```python
from build123d import *

# Parameters (mm, degrees)
SKETCH1_W           = 242
SKETCH1_H           = 13
SKETCH1_R           = 1.5
BOSS_EXTRUDE1_DEPTH = 2
CUT_EXTRUDE1_REACH  = 123.713
SKETCH2_W           = 30
SKETCH2_H           = 4
SKETCH3_W           = 242
SKETCH3_H           = 2
BOSS_EXTRUDE2_DEPTH = 15
CUT_EXTRUDE2_REACH  = 124.845
SKETCH4_R           = 1.5
FILLET1_R           = 12


with BuildPart() as part:
    # Sketch1 → Boss-Extrude1 (new body)
    with BuildSketch(Plane.XY):
        with Locations((0, -6.5)):
            Rectangle(SKETCH1_W, SKETCH1_H)
        with Locations((-114, -6.5)):
            Circle(SKETCH1_R, mode=Mode.SUBTRACT)
        with Locations((-44, -6.5)):
            Circle(SKETCH1_R, mode=Mode.SUBTRACT)
        with Locations((-24, -6.5)):
            Circle(SKETCH1_R, mode=Mode.SUBTRACT)
        with Locations((27, -6.5)):
            Circle(SKETCH1_R, mode=Mode.SUBTRACT)
        with Locations((97, -6.5)):
            Circle(SKETCH1_R, mode=Mode.SUBTRACT)
    extrude(amount=BOSS_EXTRUDE1_DEPTH)

    # Sketch2 → Cut-Extrude1 (cut, up to next)
    with BuildSketch(Plane.XY.offset(2), mode=Mode.PRIVATE) as cut_extrude1_sk1:
        with Locations((-3, -11)):
            Rectangle(SKETCH2_W, SKETCH2_H)
    cut_extrude1_tool1 = extrude(cut_extrude1_sk1.sketch, amount=-CUT_EXTRUDE1_REACH, mode=Mode.PRIVATE) & part.part
    add(cut_extrude1_tool1.solids().sort_by_distance((-3, -11, 2))[0], mode=Mode.SUBTRACT)

    # Sketch3 → Boss-Extrude2 (add)
    with BuildSketch(Plane.XY):
        with Locations((0, 1)):
            Rectangle(SKETCH3_W, SKETCH3_H)
    extrude(amount=BOSS_EXTRUDE2_DEPTH)

    # Sketch4 → Cut-Extrude2 (cut, up to next)
    with BuildSketch(Plane(origin=(0, 2, 0), x_dir=(1, 0, 0), z_dir=(0, 1, 0)), mode=Mode.PRIVATE) as cut_extrude2_sk1:
        with Locations(Location((-110, -7.5, 0), (0, 0, 270))):
            Circle(SKETCH4_R)
    cut_extrude2_tool1 = extrude(cut_extrude2_sk1.sketch, amount=-CUT_EXTRUDE2_REACH, mode=Mode.PRIVATE) & part.part
    # Sketch4 → Cut-Extrude2 (cut, up to next)
    with BuildSketch(Plane(origin=(0, 2, 0), x_dir=(1, 0, 0), z_dir=(0, 1, 0)), mode=Mode.PRIVATE) as cut_extrude2_sk2:
        with Locations(Location((-50, -7.5, 0), (0, 0, 270))):
            Circle(SKETCH4_R)
    cut_extrude2_tool2 = extrude(cut_extrude2_sk2.sketch, amount=-CUT_EXTRUDE2_REACH, mode=Mode.PRIVATE) & part.part
    # Sketch4 → Cut-Extrude2 (cut, up to next)
    with BuildSketch(Plane(origin=(0, 2, 0), x_dir=(1, 0, 0), z_dir=(0, 1, 0)), mode=Mode.PRIVATE) as cut_extrude2_sk3:
        with Locations(Location((45, -7.5, 0), (0, 0, 270))):
            Circle(SKETCH4_R)
    cut_extrude2_tool3 = extrude(cut_extrude2_sk3.sketch, amount=-CUT_EXTRUDE2_REACH, mode=Mode.PRIVATE) & part.part
    # Sketch4 → Cut-Extrude2 (cut, up to next)
    with BuildSketch(Plane(origin=(0, 2, 0), x_dir=(1, 0, 0), z_dir=(0, 1, 0)), mode=Mode.PRIVATE) as cut_extrude2_sk4:
        with Locations(Location((112, -7.5, 0), (0, 0, 270))):
            Circle(SKETCH4_R)
    cut_extrude2_tool4 = extrude(cut_extrude2_sk4.sketch, amount=-CUT_EXTRUDE2_REACH, mode=Mode.PRIVATE) & part.part
    add(cut_extrude2_tool1.solids().sort_by_distance((-110, 2, 7.5))[0], mode=Mode.SUBTRACT)
    add(cut_extrude2_tool2.solids().sort_by_distance((-50, 2, 7.5))[0], mode=Mode.SUBTRACT)
    add(cut_extrude2_tool3.solids().sort_by_distance((45, 2, 7.5))[0], mode=Mode.SUBTRACT)
    add(cut_extrude2_tool4.solids().sort_by_distance((112, 2, 7.5))[0], mode=Mode.SUBTRACT)

    # Fillet1
    fillet1_edges = [part.edges().sort_by_distance(p)[0] for p in [
        (-121, 1, 15),
        (121, 1, 15),
        (121, -13, 1),
        (-121, -13, 1),
    ]]
    fillet(fillet1_edges, radius=FILLET1_R)


solid = part.part
```
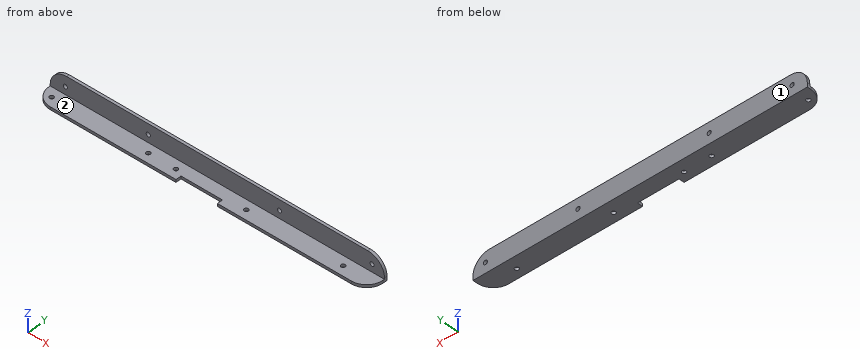
Part model, mm, in its own coordinate system. Face numbers are marked on the shaded views. A direction names the side the tool comes from. Round coordinates to 2 decimals unless told otherwise and drop trailing zeros. Write each loop counter-clockwise with the first axis right and the second up, starting at its lowest first coordinate (ties: lowest second). Pieces come first, ordered by that corner, then holes.
Item 1: Which spindle directions (+Z, -Z, +X, -X, +Y, -Y) get a long thin tool onto all of the face, cutting with end or side? Do the marked faces 1 and 2. Say none if no direction does.
Results:
face 1: +Z, -Z, +X, -X, +Y
face 2: +Z, +X, -X, -Y
Item 2: Drop flat-ended pins along their axis: pin 1 Ø1.8 at (x, y) = (27, -6.5) entering from -Z; pin 2 Ø5 at (x, y) = (1, -6) entering from +Z; pin 3 Ø1 at (y, z) = (-10, 1) entering from -X; pin 4 Ø1 at (x, z) = (30, 12.5) entering from -Y. Give the stop position or say it passes through.
Results:
pin 1: passes through
pin 2: stops at z = 2
pin 3: stops at x = -117.47
pin 4: stops at y = 0
Item 3: Probe L1, parallel to Y at x = -24, z = 0.75; L2, parallel to X at y = 0.5, z = 7.5; L3, parallel to Z at x = -110, y = 0.6. List the from-to ranges inside material, lowest first.
Results:
L1: y = -13 to -8, -5 to 2
L2: x = -120.12 to -111.5, -108.5 to -51.5, -48.5 to 43.5, 46.5 to 110.5, 113.5 to 120.12
L3: z = 0 to 6, 9 to 14.96
Item 4: Cut at B-B, the plane y = -3. Give the cut face in (x, z), plus the area to 3 significant figures.
Results:
outline: (-120.83, 0) - (120.83, 0) - (120.83, 2) - (-120.83, 2) - close
area: 483 mm2
Item 5: Cut at A-A, the plane x = -38. Give the cut face in (y, z).
Results:
outline: (-13, 0) - (2, 0) - (2, 15) - (0, 15) - (0, 2) - (-13, 2) - close
